Could you check a few things on this model? Use its own coordinates, in mm. Face numbers are marked on the shaded views. Give positions to 0.01 mm unless a question says otherwise; leave off trailing zeros. Order: outer loops, then holes, each group sorted by start corner. A loop starts at its lowest first (then second) coordinate and runs counter-clockwise, first axis right, second up. Notation, with made-up numbers: (59.5, 70) -> (96.5, 70) arc R24 cw to (96.5, 102) -> close; hole circle Ø8 at (53, 48.25). An arc over 180 degrees is marked (long way). Answer as CSV lines item,"result". Start each with the question number.
(1) I want a section at D-D (x = -874). Give the number of separate pieces and of enclosed holes in the cut face, plus the area to 3 significant figures.
(2) I want a section at A-A (x = -585.5). Please give me the cut outline in (y, z), plus the area to 3 significant figures.
(3) I need wall thicknesses on L1, parallel to Y at x = -476, z = 42; L2, parallel to Y at x = -858.5, z = 65; L3, parallel to Z at x = -852, y = -1. Which ranges of each line are inside material? Lowest first, please.
(4) We'd pull the mould along Y, two halves only. Please class the marked faces 1, 2 and 3: released by +Y, released by -Y, zero draft, split by the parting line, or undercut.
(5) I want a section at B-B (y = -40). Please give me the cut outline in (x, z), plus the area to 4 significant figures.
(6) I want a section at C-C (y = 276). Please give me the cut outline in (x, z), plus the area to 3 significant figures.
(7) Will these pins go through, and if not, where does the flat tip stop? pin 1 Ø2 at (x, z) = (-735.5, 28) entering from +Y; pin 2 Ø3 at (y, z) = (27.5, 43.5) entering from -X; pin 3 Ø24 at (x, z) = (-280, 34.5) entering from +Y; pin 4 Ø19 at (y, z) = (27, 55) entering from +X.
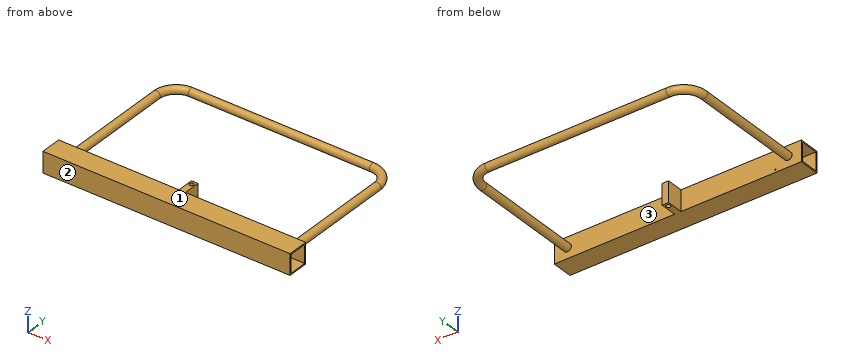
```python
from build123d import *

# Parameters (mm, degrees)
F0_W      = 80
F0_H      = 80
F0_W_2    = 70
F0_H_2    = 70
F1_DEPTH  = 952.5
F4_R      = 15
F7_W      = 63.5
F7_H      = 80
F8_DEPTH  = 12.5
F9_R      = 7.9375
F10_DEPTH = 80.001
F11_R     = 2
F12_DEPTH = 5


with BuildPart() as f1:
    # F0 (on Right) → F1 (new body)
    with BuildSketch(Plane.YZ):
        with Locations((-40, 40)):
            Rectangle(F0_W, F0_H)
        with Locations((-40, 40)):
            Rectangle(F0_W_2, F0_H_2, mode=Mode.SUBTRACT)
    extrude(amount=-F1_DEPTH)

    # F5: sweep along a path in F3
    with BuildLine(Plane.XY.offset(40)) as f5_path:
        Line((-50.8, 0), (-50.8, 431.8))
        ThreePointArc((-50.8, 431.8), (-73.1184632736, 485.6815367264), (-127, 508))
        Line((-127, 508), (-825.5, 508))
        ThreePointArc((-825.5, 508), (-879.3815367264, 485.6815367264), (-901.7, 431.8))
        Line((-901.7, 431.8), (-901.7, 0))
    # F4 (on face) → F5 (sweep)
    with BuildSketch(Plane(origin=(0, 0, 0), x_dir=(-1, 0, 0), z_dir=(0, 1, 0))):
        with Locations((50.8, 40)):
            Circle(F4_R)
    sweep(path=f5_path.line)

    # F7 (on mid) → F8 (join, symmetric)
    with BuildSketch(Plane.YZ.offset(-476.25)):
        with Locations((31.75, 40)):
            Rectangle(F7_W, F7_H)
    extrude(amount=F8_DEPTH, both=True)

    # F9 (on face) → F10 (cut, through all)
    with BuildSketch(Plane.XY.offset(80)):
        with Locations((-476.25, 47.625)):
            Circle(F9_R)
    extrude(amount=-F10_DEPTH, mode=Mode.SUBTRACT)

    # F11 (on face) → F12 (cut, through all)
    with BuildSketch(Plane(origin=(0, 0, 0), x_dir=(-1, 0, 0), z_dir=(0, 1, 0))):
        with Locations((852.5, 10)):
            Circle(F11_R)
    extrude(amount=-F12_DEPTH, mode=Mode.SUBTRACT)


solid = f1.part
```
Final values:
1,separate pieces,"2"
1,enclosed holes,"1"
1,area,"2,430 mm²"
2,outline,"(-80, 0) -> (0, 0) -> (0, 80) -> (-80, 80) -> close; circle Ø30 at (508, 40); hole (-75, 5) -> (-5, 5) -> (-5, 75) -> (-75, 75) -> close"
2,area,"2,210 mm²"
3,L1,"-80 to -75, -5 to 39.69, 55.56 to 63.5, 493.13 to 522.87"
3,L2,"-80 to -75, -5 to 0"
3,L3,"0 to 8.06, 11.94 to 80"
4,face 1,"zero draft"
4,face 2,"released by -Y"
4,face 3,"undercut"
5,outline,"(-952.5, 0) -> (0, 0) -> (0, 5) -> (-952.5, 5) -> close; (-952.5, 75) -> (0, 75) -> (0, 80) -> (-952.5, 80) -> close"
5,area,"9,525 mm²"
6,outline,"circle Ø30 at (-901.7, 40); circle Ø30 at (-50.8, 40)"
6,area,"1,410 mm²"
7,pin 1,"y = 518.2"
7,pin 2,"x = -916.57"
7,pin 3,"y = 523"
7,pin 4,"x = -36.84"
